Could you check a few things on this model? Use its own coordinates, in mm. Give positions to 0.01 mm unless a question says otherwise; leave off trailing zeros. Order: outer loops, then holes, each group sorted by start corner. A loop starts at its lowest first (then second) coordinate and runs counter-clockwise, first axis right, second up. Notation, with made-up numbers: (81.5, 65.25) -> (114.5, 65.25) arc R23 ccw to (114.5, 89.25) -> close; hole circle Ø6 at (23.5, -12.5). An arc over 180 degrees is marked (long way). Answer as CSV lines item,"result". Start each with the question number.
(1) I want a section at B-B (x = -114). Please give me the cut outline in (y, z), plus the area to 3 significant figures.
(2) I need wall thicknesses on L1, parallel to X at y = 27, z = 2.9; L2, parallel to X at y = 106, z = 3.65; L3, parallel to Y at x = -120, z = 0.5. Which ranges of each line are inside material? Lowest first, please.
(3) I want a section at D-D (x = -170.5). Please give me the cut outline in (y, z), plus the area to 3 significant figures.
(4) I want a section at A-A (z = 2.4). Please give me the cut outline in (x, y) (3 decimals), plus the area to 3 significant figures.
(5) Will these pins go through, and if not, where does the flat tip stop? pin 1 Ø2.5 at (x, z) = (-182.5, 3.5) entering from -Y; pin 2 Ø1.9 at (y, z) = (-20, 1.5) entering from +X; pin 3 Ø1.5 at (x, z) = (-178.5, 2.5) entering from +Y.
(6) I want a section at C-C (y = 32.5). Please give me the cut outline in (x, z).
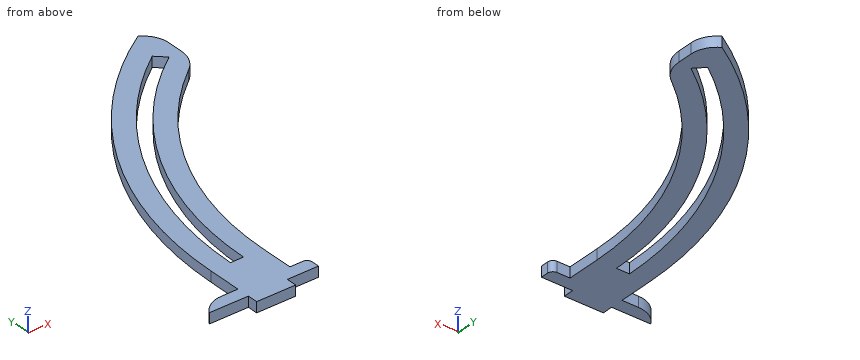
```python
from build123d import *

# Parameters (mm, degrees)
EXTRUDE_THIN2_DEPTH          = 5.08
CUT_EXTRUDE_THIN3_DEPTH      = 247.111451582
CUT_EXTRUDE_THIN3_DEPTH_BACK = 5.08
SKETCH9_W                    = 25.4
SKETCH9_H                    = 5.08
BOSS_EXTRUDE3_DEPTH          = 22.86
BOSS_EXTRUDE4_DEPTH          = 19.05
BOSS_EXTRUDE4_DEPTH_BACK     = 34.29
SKETCH10_W                   = 5.08
SKETCH10_H                   = 6.35
SKETCH11_W                   = 12.7
SKETCH11_H                   = 5.08
BOSS_EXTRUDE5_DEPTH          = 5.08
SKETCH12_W                   = 168.813467259
SKETCH12_H                   = 220.237806267
CUT_EXTRUDE1_DEPTH           = 260.928390331
SKETCH13_W                   = 5.08
SKETCH13_H                   = 30.900567514
BOSS_EXTRUDE6_DEPTH          = 6.35
FILLET2_R                    = 15.24
FILLET3_R                    = 12.7
FILLET4_R                    = 12.7
FILLET5_R                    = 2.54
BOSS_EXTRUDE14_DEPTH         = 5.08
SKETCH16_W                   = 5.08
SKETCH16_H                   = 5.08
BOSS_EXTRUDE15_DEPTH         = 6.35


with BuildPart() as part:
    # Sketch7 → Extrude-Thin2 (new body)
    with BuildSketch(Plane.XY):
        with BuildLine():
            ThreePointArc((-173.99, 0), (-123.029508859, 123.029508859), (0, 173.99))
            Line((0, 173.99), (0, 148.59))
            ThreePointArc((0, 148.59), (-105.068996617, 105.068996617), (-148.59, 0))
            Line((-148.59, 0), (-173.99, 0))
        make_face()
    extrude(amount=EXTRUDE_THIN2_DEPTH)

    # Sketch8 → Cut-Extrude-Thin3 (cut, two sides: drawn at the far end of the back side and taken through both)
    with BuildSketch(Plane.XY.offset(5.08).offset(-CUT_EXTRUDE_THIN3_DEPTH_BACK)):
        with BuildLine():
            ThreePointArc((-164.465, 0), (-116.294316768, 116.294316768), (0, 164.465))
            Line((0, 164.465), (0, 158.115))
            ThreePointArc((0, 158.115), (-111.804188707, 111.804188707), (-158.115, 0))
            Line((-158.115, 0), (-164.465, 0))
        make_face()
    extrude(amount=CUT_EXTRUDE_THIN3_DEPTH + CUT_EXTRUDE_THIN3_DEPTH_BACK, mode=Mode.SUBTRACT)


with BuildPart() as cut_extrude_thin3_piece_1:
    # of the separate pieces the step leaves, piece 1, a body of its own (cut_extrude_thin3_pieces)
    add(part.part.solids().sort_by_distance((0, 173.99, 0))[0])



with BuildPart() as cut_extrude_thin3_piece_2:
    # of the separate pieces the step leaves, piece 2, a body of its own (cut_extrude_thin3_pieces)
    add(part.part.solids().sort_by_distance((0, 158.115, 0))[0])


with BuildPart() as cut_extrude_thin3_piece_1_1:
    add(cut_extrude_thin3_piece_1.part)

    add(cut_extrude_thin3_piece_2.part)  # Boss-Extrude3 merges Cut-Extrude-Thin3 piece 2
    # Sketch9 → Boss-Extrude3 (add)
    with BuildSketch(Plane.XZ):
        with Locations((-161.29, 2.54)):
            Rectangle(SKETCH9_W, SKETCH9_H)
    extrude(amount=BOSS_EXTRUDE3_DEPTH)

    # Sketch10 → Boss-Extrude4 (add, two sides: drawn at the far end of the back side and taken through both)
    with BuildSketch(Plane.ZY.offset(173.99).offset(-BOSS_EXTRUDE4_DEPTH_BACK)):
        with Locations((2.54, -19.685)):
            Rectangle(SKETCH10_W, SKETCH10_H)
    extrude(amount=BOSS_EXTRUDE4_DEPTH + BOSS_EXTRUDE4_DEPTH_BACK)

    # Sketch11 → Boss-Extrude5 (add)
    with BuildSketch(Plane.XZ.offset(22.86)):
        with Locations((-161.29, 2.54)):
            Rectangle(SKETCH11_W, SKETCH11_H)
    extrude(amount=BOSS_EXTRUDE5_DEPTH)

    # Sketch12 → Cut-Extrude1 (cut, through all)
    with BuildSketch(Plane.XY.offset(5.08)):
        with Locations((-7.025506372, 87.258903133)):
            Rectangle(SKETCH12_W, SKETCH12_H)
    extrude(amount=-CUT_EXTRUDE1_DEPTH, mode=Mode.SUBTRACT)

    # Sketch13 → Boss-Extrude6 (add)
    with BuildSketch(Plane(origin=(-91.432240001, 0, 0), x_dir=(0, 0, -1), z_dir=(1, 0, 0))):
        with Locations((-2.54, 132.578988985)):
            Rectangle(SKETCH13_W, SKETCH13_H)
    extrude(amount=BOSS_EXTRUDE6_DEPTH)

    # Fillet2
    # the kernel refuses this fillet: 15.24 mm, written as the material it takes off along each edge
    with BuildSketch(Plane(origin=(-85.082240001, 117.128705228, -30.946072045), x_dir=(-1, 0, 0), z_dir=(0, 0, 1))) as fillet2_piece_1:
        with BuildLine():
            CenterArc((15.24, -12.378428818), FILLET2_R, 125.685334713, 54.314665287)
            Line((0, -12.378428818), (-0.3048, -12.378428818))
            Line((-0.3048, -12.378428818), (-0.3048, 0))
            Line((-0.3048, 0), (0, 0.3048))
            ThreePointArc((0, 0.3048), (3.175, 0.3048), (6.1722, 0.247568576))
            Line((6.1722, 0.247568576), (6.35, 0))
        make_face()
    extrude(amount=66.97214409, mode=Mode.SUBTRACT)

    # Fillet3
    # the kernel refuses this fillet: 12.7 mm, written as the material it takes off along each edge
    with BuildSketch(Plane(origin=(-85.082240001, 148.029272742, 32.57630657), x_dir=(0, -1, 0), z_dir=(0, 0, -1))) as fillet3_piece_1:
        with BuildLine():
            CenterArc((10.998522628, 12.7), FILLET3_R, 210, 60)
            Line((0, 6.35), (-0.219970453, 6.223))
            ThreePointArc((-0.219970453, 6.223), (-0.254, 3.175), (-0.254, 0))
            Line((-0.254, 0), (0, -0.254))
            Line((0, -0.254), (10.998522628, -0.254))
            Line((10.998522628, -0.254), (10.998522628, 0))
        make_face()
    extrude(amount=60.07261314, mode=Mode.SUBTRACT)

    # Fillet4
    # the kernel refuses this fillet: 12.7 mm, written as the material it takes off along each edge
    with BuildSketch(Plane(origin=(-193.04, -16.51, 32.57630657), x_dir=(1, 0, 0), z_dir=(0, 0, -1))) as fillet4_piece_1:
        with BuildLine():
            CenterArc((10.998522628, 12.7), FILLET4_R, 210, 60)
            Line((0, 6.35), (-0.219970453, 6.223))
            ThreePointArc((-0.219970453, 6.223), (-0.254, 3.175), (-0.254, 0))
            Line((-0.254, 0), (0, -0.254))
            Line((0, -0.254), (10.998522628, -0.254))
            Line((10.998522628, -0.254), (10.998522628, 0))
        make_face()
    extrude(amount=60.07261314, mode=Mode.SUBTRACT)

    # Fillet5
    fillet5_edges = [cut_extrude_thin3_piece_1_1.edges().sort_by_distance(p)[0] for p in [
        (-139.7, -16.51, 2.54),
    ]]
    fillet(fillet5_edges, radius=FILLET5_R)

    # Sketch15 → Boss-Extrude14 (add)
    with BuildSketch(Plane.XY):
        Polygon((-91.432240001, 128.998057014), (-96.042586765, 133.508642988), (-90.011669105, 142.911064998), (-86.217351324, 133.783124359), align=None)
    extrude(amount=BOSS_EXTRUDE14_DEPTH)

    # Sketch16 → Boss-Extrude15 (add)
    with BuildSketch(Plane.ZY.offset(167.64)):
        with Locations((2.54, -25.4)):
            Rectangle(SKETCH16_W, SKETCH16_H)
    extrude(amount=BOSS_EXTRUDE15_DEPTH)


solid = cut_extrude_thin3_piece_1_1.part
```
Final values:
1,outline,"(95.3, 0) -> (109.56, 0) -> (109.56, 5.08) -> (95.3, 5.08) -> close; (118.54, 0) -> (131.44, 0) -> (131.44, 5.08) -> (118.54, 5.08) -> close"
1,area,"138 mm²"
2,L1,"-171.88 to -162.23, -155.79 to -146.12"
2,L2,"-137.97 to -125.75, -117.32 to -104.13"
2,L3,"87.63 to 102.96, 112.47 to 125.99"
3,outline,"(-27.94, 0) -> (34.67, 0) -> (34.67, 5.08) -> (-27.94, 5.08) -> close"
3,area,"318 mm²"
4,outline,"(-193.04, -22.86) -> (-173.99, -22.86) -> (-173.99, -27.94) -> (-154.94, -27.94) -> (-154.94, -22.86) -> (-139.7, -22.86) -> (-139.7, -19.05) arc R2.54 ccw to (-142.24, -16.51) -> (-148.59, -16.51) -> (-148.59, 0) arc R148.59 cw to (-91.432, 117.129) arc R15.24 ccw to (-85.082, 129.507) -> (-85.082, 137.031) arc R12.7 ccw to (-91.432, 148.029) arc R173.99 ccw to (-173.99, 0) -> (-173.99, -16.51) -> (-182.041, -16.51) arc R12.7 ccw to start; hole (-164.465, 0) -> (-158.115, 0) arc R158.115 cw to (-91.432, 128.998) -> (-96.043, 133.509) arc R164.465 ccw to start"
4,area,"3,980 mm²"
5,pin 1,"y = -22.86"
5,pin 2,"x = -139.7"
5,pin 3,"y = -16.51"
6,outline,"(-170.93, 0) -> (-161.22, 0) -> (-161.22, 5.08) -> (-170.93, 5.08) -> close; (-154.74, 0) -> (-144.99, 0) -> (-144.99, 5.08) -> (-154.74, 5.08) -> close"
